Design review of the part built by this model. Coordinates are the model's own, in mm. A direction names the side the tool comes from. Give positions to 0.01 mm unless a question says otherwise; leave off trailing zeros. Order: outer loops, then holes, each group sorted by start corner. A loop starts at its lowest first (then second) coordinate and runs counter-clockwise, first axis right, second up. Notation, with made-up numbers: M 14,-12.75 L 71,-12.75 A31 ccw 71,24.25 Z; hole C 13,80 d1. An arc over 180 degrees is marked long. Answer as a JSON object with one key per item and string values.
from build123d import *

# Parameters (mm, degrees)
SKETCH1_W            = 10
SKETCH1_H            = 8
BOSS_EXTRUDE1_DEPTH  = 3
CUT_EXTRUDE1_REACH   = 15.153
LPATTERN2_COUNT      = 3
LPATTERN2_PITCH      = 3
LPATTERN2_COUNT_DIR2 = 3
LPATTERN2_PITCH_DIR2 = 1.732050808


with BuildPart() as part:
    # Sketch1 → Boss-Extrude1 (new body)
    with BuildSketch(Plane(origin=(0, 0, 0), x_dir=(1, 0, 0), z_dir=(0, 1, 0))):
        with Locations((5, 4)):
            Rectangle(SKETCH1_W, SKETCH1_H)
    extrude(amount=BOSS_EXTRUDE1_DEPTH)

    # Sketch2 → Cut-Extrude1 (cut, up to next)
    with BuildSketch(Plane(origin=(0, 3, 0), x_dir=(1, 0, 0), z_dir=(0, 1, 0)), mode=Mode.PRIVATE) as cut_extrude1_sk1:
        Polygon((2.076794919, 1.291025404), (1.620096189, 2.082050808), (0.70669873, 2.082050808), (0.25, 1.291025404), (0.70669873, 0.5), (1.620096189, 0.5), align=None)
    cut_extrude1_tool1 = extrude(cut_extrude1_sk1.sketch, amount=-CUT_EXTRUDE1_REACH, mode=Mode.PRIVATE) & part.part
    # Sketch2 → Cut-Extrude1 (cut, up to next)
    with BuildSketch(Plane(origin=(0, 3, 0), x_dir=(1, 0, 0), z_dir=(0, 1, 0)), mode=Mode.PRIVATE) as cut_extrude1_sk2:
        Polygon((3.576794919, 2.157050808), (3.120096189, 2.948076211), (2.20669873, 2.948076211), (1.75, 2.157050808), (2.20669873, 1.366025404), (3.120096189, 1.366025404), align=None)
    cut_extrude1_tool2 = extrude(cut_extrude1_sk2.sketch, amount=-CUT_EXTRUDE1_REACH, mode=Mode.PRIVATE) & part.part
    cut_extrude1_1 = cut_extrude1_tool1.solids().sort_by_distance((1.163397, 3, -1.291025))[0]
    add(cut_extrude1_1, mode=Mode.SUBTRACT)
    cut_extrude1_2 = cut_extrude1_tool2.solids().sort_by_distance((2.663397, 3, -2.157051))[0]
    add(cut_extrude1_2, mode=Mode.SUBTRACT)
    cut_extrude1 = cut_extrude1_1 + cut_extrude1_2  # Cut-Extrude1 as one shape, for the pattern or mirror that repeats it

    # LPattern2: Cut-Extrude1 3 × 3
    with Locations(*[(i * LPATTERN2_PITCH, 0, -j * LPATTERN2_PITCH_DIR2) for i in range(LPATTERN2_COUNT) for j in range(LPATTERN2_COUNT_DIR2) if (i, j) != (0, 0)]):
        add(cut_extrude1, mode=Mode.SUBTRACT)


solid = part.part
(1) We need section B-B (z = -3.5). Write out the cut boundary in (x, y).
Checked values:
{"outline": "M 0,0 L 0.53,0 L 0.53,3 L 0,3 Z; M 1.8,0 L 1.97,0 L 1.97,3 L 1.8,3 Z; M 3.35,0 L 3.53,0 L 3.53,3 L 3.35,3 Z; M 4.8,0 L 4.97,0 L 4.97,3 L 4.8,3 Z; M 6.35,0 L 6.53,0 L 6.53,3 L 6.35,3 Z; M 7.8,0 L 7.97,0 L 7.97,3 L 7.8,3 Z; M 9.35,0 L 10,0 L 10,3 L 9.35,3 Z"}
(2) Tool access review of faces 4 (the flat face through (8.7, 1.5, -4.68)), 5 (the flat face through (5, 1, 0)): name each direction out of +Z, -Z, +X, -X, +Y, -Y from which nothing blocks a thin tool from reaching the whole face with its end or side.
Checked values:
{"face 4": "+Y, -Y", "face 5": "+Z, +X, -X, +Y, -Y"}
(3) We need section C-C (y = 1.5). Count the separate pieces of the cut face and the enclosed holes in it, plus the area to 3 significant figures.
Checked values:
{"separate pieces": "1", "enclosed holes": "18", "area": "41.0 mm^2"}
(4) To check wall thickness, follow L1, parallel to Z at x = 2.25, y = 0.65; L2, parallel to X at y = 0.7, z = -5.75; L3, parallel to X at y = 1.65, z = -1. State the ranges of each line that lie inside material, in increasing order. Write a range as from..to.
Checked values:
{"L1": "z = -8..-6.41, -4.83..-4.68, -3.1..-2.95, -1.37..0", "L2": "x = 0..1.82, 3.5..4.82, 6.5..7.82, 9.5..10", "L3": "x = 0..0.42, 1.91..3.42, 4.91..6.42, 7.91..10"}
(5) Draft analysis for pull direction X (two halves, no side actions). For faces 1 (the flat face through (4, 0, -6)), 2 (the flat face through (0, 1, -4)), 3 (the flat face through (7, 2, -0.5)), state which applies: +X half, -X half, draft (parallel to the pull), parting line (faces both ways), or undercut.
Checked values:
{"face 1": "draft", "face 2": "-X half", "face 3": "undercut"}
(6) We need section A-A (x = 3). Write out the cut boundary in (y, z).
Checked values:
{"outline": "M 0,-8 L 3,-8 L 3,-6.41 L 0,-6.41 Z; M 0,-4.83 L 3,-4.83 L 3,-4.68 L 0,-4.68 Z; M 0,-3.1 L 3,-3.1 L 3,-2.95 L 0,-2.95 Z; M 0,-1.37 L 3,-1.37 L 3,0 L 0,0 Z"}
